Can you work these out from the model? Positions are in its coordinate system, mm. Face numbers are marked on the shaded views. A direction names the side the tool comes from. Give positions to 0.01 mm unless a question says otherwise; leave off trailing zeros. Write each loop counter-clockwise with the first axis right and the second up, starting at its lowest first coordinate (ties: lowest second). Pieces come first, ordered by that corner, then holes.
from build123d import *

# Parameters (mm, degrees)
F0_W      = 500
F0_H      = 500
F1_DEPTH  = 15
F2_W      = 15
F2_H      = 500
F3_DEPTH  = 1200
F5_DEPTH  = 500
F6_W      = 500
F6_H      = 500
F7_DEPTH  = 15
F8_W      = 500
F8_H      = 250
F9_DEPTH  = 120
F10_W     = 470
F10_H     = 220
F11_DEPTH = 105
F12_R     = 10
F13_DEPTH = 25
F15_DEPTH = 25
F17_DEPTH = 25
F19_DEPTH = 500


with BuildPart() as f1:
    # F0 (on Top) → F1 (new body)
    with BuildSketch(Plane.XY):
        Rectangle(F0_W, F0_H)
    extrude(amount=F1_DEPTH)

    # F2 (on face) → F3 (join)
    with BuildSketch(Plane.XY.offset(15)):
        with Locations((-242.5, 0)):
            Rectangle(F2_W, F2_H)
        with Locations((242.5, 0)):
            Rectangle(F2_W, F2_H)
    extrude(amount=F3_DEPTH)

    # F4 (on face) → F5 (cut)
    with BuildSketch(Plane(origin=(-250, 0, 0), x_dir=(0, -1, 0), z_dir=(-1, 0, 0))):
        with BuildLine():
            Line((250, 108.3225146088), (250, 1169.652935098))
            Line((250, 1169.652935098), (124.1641795165, 1088.1852527777))
            ThreePointArc((124.1641795165, 1088.1852527777), (90.6620527914, 1052.0193626432), (78.5102322698, 1004.241780428))
            Line((78.5102322698, 1004.241780428), (78.5102322698, 341.1126717917))
            ThreePointArc((78.5102322698, 341.1126717917), (84.9402448732, 305.8329685815), (103.4033814418, 275.090244097))
            Line((103.4033814418, 275.090244097), (250, 108.3225146088))
        make_face()
    extrude(amount=-F5_DEPTH, mode=Mode.SUBTRACT)

    # F6 (on face) → F7 (join)
    with BuildSketch(Plane.XY.offset(1215)):
        Rectangle(F6_W, F6_H)
    extrude(amount=F7_DEPTH)

    # F8 (on face) → F9 (join)
    with BuildSketch(Plane.XY.offset(1230)):
        with Locations((0, 125)):
            Rectangle(F8_W, F8_H)
    extrude(amount=F9_DEPTH)

    # F10 (on face) → F11 (cut)
    with BuildSketch(Plane.XY.offset(1350)):
        with Locations((0, 125)):
            Rectangle(F10_W, F10_H)
    extrude(amount=-F11_DEPTH, mode=Mode.SUBTRACT)

    # F12 (on face) → F13 (cut)
    with BuildSketch(Plane.XY.offset(1230)):
        with Locations((-210.25, -235)):
            Circle(F12_R)
        with Locations((-185.5, -235)):
            Circle(F12_R)
        with Locations((-160.75, -235)):
            Circle(F12_R)
        with Locations((-136, -235)):
            Circle(F12_R)
        with Locations((-111.25, -235)):
            Circle(F12_R)
        with Locations((-86.5, -235)):
            Circle(F12_R)
        with Locations((-61.75, -235)):
            Circle(F12_R)
        with Locations((-37, -235)):
            Circle(F12_R)
        with Locations((-12.25, -235)):
            Circle(F12_R)
        with Locations((12.5, -235)):
            Circle(F12_R)
        with Locations((37.25, -235)):
            Circle(F12_R)
        with Locations((62, -235)):
            Circle(F12_R)
        with Locations((86.75, -235)):
            Circle(F12_R)
        with Locations((111.5, -235)):
            Circle(F12_R)
        with Locations((136.25, -235)):
            Circle(F12_R)
        with Locations((161, -235)):
            Circle(F12_R)
        with Locations((185.75, -235)):
            Circle(F12_R)
        with Locations((210.5, -235)):
            Circle(F12_R)
        with Locations((-210.2958800694, -210.5000429588)):
            Circle(F12_R)
        with Locations((-210.3417601387, -186.0000859177)):
            Circle(F12_R)
        with Locations((-210.3876402081, -161.5001288765)):
            Circle(F12_R)
        with Locations((-210.4335202775, -137.0001718353)):
            Circle(F12_R)
        with Locations((-210.4794003468, -112.5002147941)):
            Circle(F12_R)
        with Locations((-210.5252804162, -88.000257753)):
            Circle(F12_R)
        with Locations((-210.5711604856, -63.5003007118)):
            Circle(F12_R)
        with Locations((-210.6170405549, -39.0003436706)):
            Circle(F12_R)
        with Locations((-210.6629206243, -14.5003866295)):
            Circle(F12_R)
        with Locations((210.4541199306, -210.5000429588)):
            Circle(F12_R)
        with Locations((210.4082398613, -186.0000859177)):
            Circle(F12_R)
        with Locations((210.3623597919, -161.5001288765)):
            Circle(F12_R)
        with Locations((210.3164797225, -137.0001718353)):
            Circle(F12_R)
        with Locations((210.2705996532, -112.5002147941)):
            Circle(F12_R)
        with Locations((210.2247195838, -88.000257753)):
            Circle(F12_R)
        with Locations((210.1788395144, -63.5003007118)):
            Circle(F12_R)
        with Locations((210.1329594451, -39.0003436706)):
            Circle(F12_R)
        with Locations((210.0870793757, -14.5003866295)):
            Circle(F12_R)
    extrude(amount=-F13_DEPTH, mode=Mode.SUBTRACT)

    # F14 (on face) → F15 (cut)
    with BuildSketch(Plane(origin=(-250, 0, 0), x_dir=(0, -1, 0), z_dir=(-1, 0, 0))):
        Polygon((0, 301.9825816154), (-200.6096243858, 60.1997859776), (184.8411858082, 60.1997859776), align=None)
        Polygon((-200.6096243858, 545.617259301), (-200.6096243858, 193.3555305004), (20.2688685386, 459.5671825039), (20.2688685386, 811.8289113045), align=None)
        Polygon((-200.6096243858, 903.4412830945), (-200.6096243858, 697.9457139969), (20.2688685386, 964.1573660004), (20.2688685386, 1169.652935098), align=None)
    extrude(amount=-F15_DEPTH, mode=Mode.SUBTRACT)

    # F16 (on face) → F17 (cut)
    with BuildSketch(Plane.YZ.offset(250)):
        Polygon((200.6096243858, 903.4412830945), (-20.2688685386, 1169.652935098), (-20.2688685386, 964.1573660004), (200.6096243858, 697.9457139969), align=None)
        Polygon((200.6096243858, 545.617259301), (-20.2688685386, 811.8289113045), (-20.2688685386, 459.5671825039), (200.6096243858, 193.3555305004), align=None)
        Polygon((200.6096243858, 60.1997859776), (0, 301.9825816154), (-184.8411858082, 60.1997859776), align=None)
    extrude(amount=-F17_DEPTH, mode=Mode.SUBTRACT)

    # F18 (on face) → F19 (join)
    with BuildSketch(Plane(origin=(-250, 0, 0), x_dir=(0, -1, 0), z_dir=(-1, 0, 0))):
        with BuildLine():
            add(Edge.make_bspline(
                [(53.9202547284, 1096.9846327727), (54.7732887858, 1098.0347093312), (55.4434477794, 1099.2897070818), (56.4611232834, 1100.4414988147)],
                knots=[0, 0, 0, 0, 0.0893664626, 0.0893664626, 0.0893664626, 0.0893664626], degree=3))
            ThreePointArc((53.9202547284, 1096.9846327727), (58.7459698854, 1074.3814357408), (81.7806412913, 1076.2777363651))
            add(Edge.make_bspline(
                [(81.7806412913, 1076.2777363651), (82.0130700174, 1076.5925295791), (82.3047431486, 1076.8573193246), (82.629787133, 1077.224659717)],
                knots=[0, 0, 0, 0, 0.0708567707, 0.0708567707, 0.0708567707, 0.0708567707], degree=3))
            ThreePointArc((82.629787133, 1077.224659717), (83.3571621202, 1078.1603319134), (84.0195396019, 1079.1430897184))
            add(Edge.make_bspline(
                [(84.0195396019, 1079.1430897183), (84.4659025247, 1079.8776865412), (84.8451263222, 1080.6456217553), (85.1639807224, 1081.2907218933)],
                knots=[0.1675578427, 0.1675578427, 0.1675578427, 0.1675578427, 0.2655687466, 0.2655687466, 0.2655687466, 0.2655687466], degree=3))
            ThreePointArc((85.1639807224, 1081.2907218933), (86.3005857895, 1084.7786499445), (86.6850861658, 1088.4268923473))
            ThreePointArc((86.6850861658, 1088.4268923473), (79.4162565109, 1102.6245383975), (63.6481543522, 1105.0278678033))
            add(Edge.make_bspline(
                [(60.3427219255, 1103.5286337913), (61.44755319, 1104.15284537), (62.4027767886, 1104.4920782739), (63.6481543522, 1105.0278678033)],
                knots=[0.1854516751, 0.1854516751, 0.1854516751, 0.1854516751, 0.2676496457, 0.2676496457, 0.2676496457, 0.2676496457], degree=3))
            ThreePointArc((60.3427219255, 1103.5286337913), (58.2920050139, 1102.1232708109), (56.4611232834, 1100.4414988147))
        make_face()
        with BuildLine():
            ThreePointArc((56.4611232834, 1100.4414988147), (55.0843545331, 1098.7912238464), (53.9202547284, 1096.9846327727))
            add(Edge.make_bspline(
                [(53.9202547284, 1096.9846327727), (54.7732887858, 1098.0347093312), (55.4434477794, 1099.2897070818), (56.4611232834, 1100.4414988147)],
                knots=[0, 0, 0, 0, 0.0893664626, 0.0893664626, 0.0893664626, 0.0893664626], degree=3))
        make_face()
        with BuildLine():
            add(Edge.make_bspline(
                [(81.7806412913, 1076.2777363651), (82.0130700174, 1076.5925295791), (82.3047431486, 1076.8573193246), (82.629787133, 1077.224659717)],
                knots=[0, 0, 0, 0, 0.0708567707, 0.0708567707, 0.0708567707, 0.0708567707], degree=3))
            ThreePointArc((81.7806412913, 1076.2777363651), (82.2138198073, 1076.7434810433), (82.629787133, 1077.224659717))
        make_face()
        with BuildLine():
            add(Edge.make_bspline(
                [(56.4611232834, 1100.4414988147), (57.5553096742, 1101.6798845617), (59.0512308325, 1102.798962465), (60.3427219255, 1103.5286337913)],
                knots=[0.0893664626, 0.0893664626, 0.0893664626, 0.0893664626, 0.1854516751, 0.1854516751, 0.1854516751, 0.1854516751], degree=3))
            ThreePointArc((56.4611232834, 1100.4414988147), (58.2920050139, 1102.1232708109), (60.3427219255, 1103.5286337913))
        make_face()
        with BuildLine():
            ThreePointArc((63.6481543522, 1105.0278678033), (61.956464969, 1104.3641767958), (60.3427219255, 1103.5286337913))
            add(Edge.make_bspline(
                [(60.3427219255, 1103.5286337913), (61.44755319, 1104.15284537), (62.4027767886, 1104.4920782739), (63.6481543522, 1105.0278678033)],
                knots=[0.1854516751, 0.1854516751, 0.1854516751, 0.1854516751, 0.2676496457, 0.2676496457, 0.2676496457, 0.2676496457], degree=3))
        make_face()
        with BuildLine():
            add(Edge.make_bspline(
                [(84.0195396019, 1079.1430897183), (84.4659025247, 1079.8776865412), (84.8451263222, 1080.6456217553), (85.1639807224, 1081.2907218933)],
                knots=[0.1675578427, 0.1675578427, 0.1675578427, 0.1675578427, 0.2655687466, 0.2655687466, 0.2655687466, 0.2655687466], degree=3))
            ThreePointArc((84.0195396019, 1079.1430897184), (84.6291363023, 1080.1969886188), (85.1639807224, 1081.2907218933))
        make_face()
    extrude(amount=-F19_DEPTH)


solid = f1.part
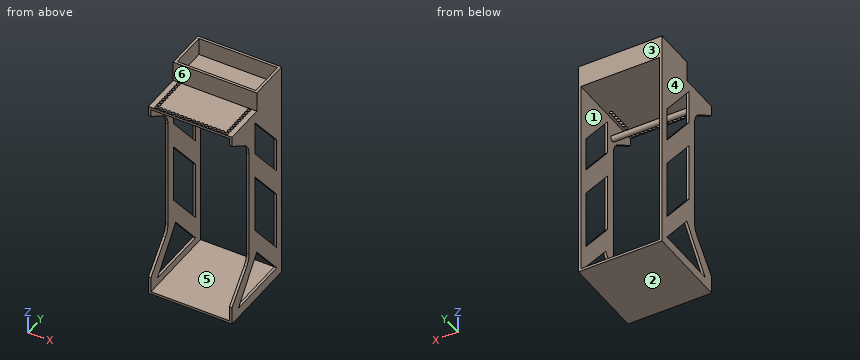
(1) For the marked faces 4, 5 and 6, which set-ups out of +Z, -Z, +X, -X, +Y, -Y let a thin tool reach every point of the face, with its end or its side?
Returned:
face 4: +Z, -Z, -X, +Y, -Y
face 5: +Y, -Y
face 6: +Z, +X, -X, -Y
(2) If we mould it in two halves opening along Z, with no side actions, what happens to the marked faces 1, 2 and 3? For each: +Z half, -Z half, draft (parallel to the pull), parting line (faces both ways), or undercut.
Returned:
face 1: undercut
face 2: -Z half
face 3: draft
(3) Imagine slicing it at B-B, the plane z = 161. Write out the boundary of the cut face in (x, y), plus the area to 3 significant figures.
Returned:
outline: (-250, -203.69) - (-235, -203.69) - (-235, -107.78) - (-250, -107.78) - close; (-250, 116.97) - (-235, 116.97) - (-235, 250) - (-250, 250) - close; (235, -203.69) - (250, -203.69) - (250, -107.78) - (235, -107.78) - close; (235, 116.97) - (250, 116.97) - (250, 250) - (235, 250) - close
area: 6,870 mm2
(4) Imagine slicing it at A-A, the plane z = 520.5. Write out the boundary of the cut face in (x, y), plus the area to 3 significant figures.
Returned:
outline: (-250, -78.51) - (-235, -78.51) - (-235, -20.27) - (-250, -20.27) - close; (-250, 200.61) - (-235, 200.61) - (-235, 250) - (-250, 250) - close; (235, -78.51) - (250, -78.51) - (250, -20.27) - (235, -20.27) - close; (235, 200.61) - (250, 200.61) - (250, 250) - (235, 250) - close
area: 3,230 mm2
(5) If I drill on L1, parallel to Z at x = 134, y = 120.5; L2, parallel to X at y = 75.5, z = 842.5; L3, parallel to Z at x = -157, y = -69.5, over which ranges is the centre line in solid material (lowest first)?
Returned:
L1: z = 0 to 15, 1215 to 1245
L2: x = -250 to -235, 235 to 250
L3: z = 0 to 15, 1070.93 to 1105.92, 1215 to 1230
(6) Will these pins go through, and if not, where does the flat tip stop? P1, Ø12, axis at x = 245.5, z = 786, coming from the -Y side; P2, Ø18, axis at x = -210.57, y = -63.5, coming from the +Z side; P3, Ø18, axis at x = 136.25, y = -235, coming from the +Z side.
Returned:
P1: stops at y = -78.51
P2: stops at z = 1105.93
P3: stops at z = 15
